Part model, mm, in its own coordinate system. A direction names the side the tool comes from. Give positions to 0.01 mm unless a question says otherwise; leave off trailing zeros. Write each loop counter-clockwise with the first axis right and the second up, starting at its lowest first coordinate (ties: lowest second). Pieces come first, ordered by that corner, then holes.
from build123d import *

# Parameters (mm, degrees)
CUT_EXTRUDE1_START = 11
CUT_EXTRUDE1_DEPTH = 92.225241501


with BuildPart() as part:
    # Sketch1 → Revolve1 (revolve)
    with BuildSketch(Plane(origin=(0, 0, 0), x_dir=(0, 0, -1), z_dir=(1, 0, 0)), mode=Mode.PRIVATE) as revolve1_sk:
        Polygon((0, 15), (70, 15), (70, 12.5), (100, 12.5), (100, 0), (-30, 0), (-30, 12.5), (0, 12.5), align=None)
    revolve(revolve1_sk.sketch.rotate(Axis((0, 0, 91.723358082), (0, 0, -1)), 90), axis=Axis((0, 0, 91.723358082), (0, 0, -1)))

    # Sketch2 → Cut-Extrude1 (cut, through all)
    with BuildSketch(Plane(origin=(0, 0, 0), x_dir=(1, 0, 0), z_dir=(0, 1, 0)).offset(CUT_EXTRUDE1_START)):
        with BuildLine():
            Line((4, 46), (4, 24))
            ThreePointArc((4, 24), (0, 20), (-4, 24))
            Line((-4, 24), (-4, 46))
            ThreePointArc((-4, 46), (0, 50), (4, 46))
        make_face()
    extrude(amount=CUT_EXTRUDE1_DEPTH, mode=Mode.SUBTRACT)


solid = part.part
1) 3-axis set-ups, long thin cutter, end or side, ignore diameter. For faces 5 (the cylindrical face through (11.923, -3.755, 14.79)), 6 (the flat face through (-3.4, -12.3, -70)), 7 (the cylindrical face through (8.06, -12.65, -35.49)), 8 (the cylindrical face through (0, 13, -50)): which of +Z, -Z, +X, -X, +Y, -Y reach the whole face in a straight line?
Check result:
face 5: +Z
face 6: -Z
face 7: +Z, -Z
face 8: +Y
2) Flat gauge pins, fed straight in: P1, Ø2, axis at y = 9, z = -63, coming from the -X side; P2, Ø9, axis at x = 0.5, z = -42, coming from the +Y side; P3, Ø1.5, axis at y = 12, z = 16.5, coming from the +X side. Where does each tip first touch, or does it go through?
Check result:
P1: stops at x = -12.69
P2: stops at y = 14.46
P3: stops at x = 5.45
3) Saw through at D-D (y = 6.5). Write the cut outline in (x, z), and give its area (3 significant figures).
Check result:
outline: (-13.52, -70) - (-10.68, -70) - (-10.68, -100) - (10.68, -100) - (10.68, -70) - (13.52, -70) - (13.52, 0) - (10.68, 0) - (10.68, 30) - (-10.68, 30) - (-10.68, 0) - (-13.52, 0) - close
area: 3,170 mm2
4) Saw through at B-B (x = 0). Write the cut outline in (y, z).
Check result:
outline: (-15, -70) - (-12.5, -70) - (-12.5, -100) - (12.5, -100) - (12.5, -70) - (15, -70) - (15, -50) - (11, -50) - (11, -20) - (15, -20) - (15, 0) - (12.5, 0) - (12.5, 30) - (-12.5, 30) - (-12.5, 0) - (-15, 0) - close
5) Mould opens along Z. For faces 1 (the flat face through (0, 11, -35)), 2 (the flat face through (0, 0, 30)), 3 (the flat face through (0, 0, -100)), 4 (the flat face through (-4, 13, -35)) say: +Z half, -Z half, draft (parallel to the pull), parting line (faces both ways), or undercut.
Check result:
face 1: undercut
face 2: +Z half
face 3: -Z half
face 4: undercut
6) Saw through at C-C (z = 11). Write the cut outline in (x, y).
Check result:
outline: circle Ø25 at (0, 0)
7) Drill centre lines: L1, parallel to Z at x = -12, y = -4; L2, parallel to Z at x = -1.5, y = 12.5; L3, parallel to Y at x = 3.5, z = -32.5. Where is each one in solid material? Low to high.
Check result:
L1: z = -70 to 0
L2: z = -70 to -49.71, -20.29 to 0
L3: y = -14.59 to 11
8) Saw through at A-A (y = 0). Write the cut outline in (x, z), and give its area (3 significant figures).
Check result:
outline: (-15, -70) - (-12.5, -70) - (-12.5, -100) - (12.5, -100) - (12.5, -70) - (15, -70) - (15, 0) - (12.5, 0) - (12.5, 30) - (-12.5, 30) - (-12.5, 0) - (-15, 0) - close
area: 3,600 mm2
